Geometry: final body of the model. Coordinates: model frame, mm. Face numbers are marked on the shaded views. A direction names the side the tool comes from. Coordinates: 2 decimals unless noted, no trailing zeros. Order: outer loops, then holes, each group sorted by start corner. A loop starts at its lowest first (then second) coordinate and runs counter-clockwise, first axis right, second up. Notation, with made-up numbers: (45.25, 70) - (66.25, 70) arc R29 ccw to (66.25, 99) - close; hole circle Ø2 at (-25, 39). An arc over 180 degrees is marked (long way). Use a Markdown table: item, result. Add a question column.
```python
from build123d import *

# Parameters (mm, degrees)
EXTRUDE_1_DEPTH     = 5
SKETCH_2_R          = 5
CUT_EXTRUDE_1_DEPTH = 32.721443851
SKETCH_3_W          = 35
SKETCH_3_H          = 35
EXTRUDE_2_DEPTH     = 5
FILLET_1_R          = 10
SKETCH_4_R          = 5
CUT_EXTRUDE_2_DEPTH = 52.780787943


with BuildPart() as part:
    # 草图1 → 凸台-拉伸1 (new body)
    with BuildSketch(Plane.XY):
        with BuildLine():
            Line((0, 20), (0, -20))
            ThreePointArc((0, -20), (-7.5, -27.5), (-15, -20))
            Line((-15, -20), (-15, 20))
            ThreePointArc((-15, 20), (-7.5, 27.5), (0, 20))
        make_face()
    extrude(amount=EXTRUDE_1_DEPTH)

    # 草图2 → 切除-拉伸1 (cut, through all)
    with BuildSketch(Plane.XY.offset(5)):
        with Locations((-7.5, 20)):
            Circle(SKETCH_2_R)
        with Locations((-7.5, -20)):
            Circle(SKETCH_2_R)
    extrude(amount=-CUT_EXTRUDE_1_DEPTH, mode=Mode.SUBTRACT)

    # 草图3 → 凸台-拉伸2 (add, symmetric)
    with BuildSketch(Plane(origin=(0, 0, 0), x_dir=(1, 0, 0), z_dir=(0, 1, 0))):
        with Locations((17.5, -2.5)):
            Rectangle(SKETCH_3_W, SKETCH_3_H)
    extrude(amount=EXTRUDE_2_DEPTH, both=True)

    # 圆角1
    fillet_1_edges = [part.edges().sort_by_distance(p)[0] for p in [
        (0, 0, -15),
        (0, 0, 20),
        (35, 0, 20),
        (35, 0, -15),
    ]]
    fillet(fillet_1_edges, radius=FILLET_1_R)

    # 草图4 → 切除-拉伸2 (cut, through all)
    with BuildSketch(Plane(origin=(0, 5, 0), x_dir=(1, 0, 0), z_dir=(0, 1, 0))):
        with Locations(Location((17.5, -2.5, 0), (0, 0, 270))):
            Circle(SKETCH_4_R)
    extrude(amount=-CUT_EXTRUDE_2_DEPTH, mode=Mode.SUBTRACT)


solid = part.part
```
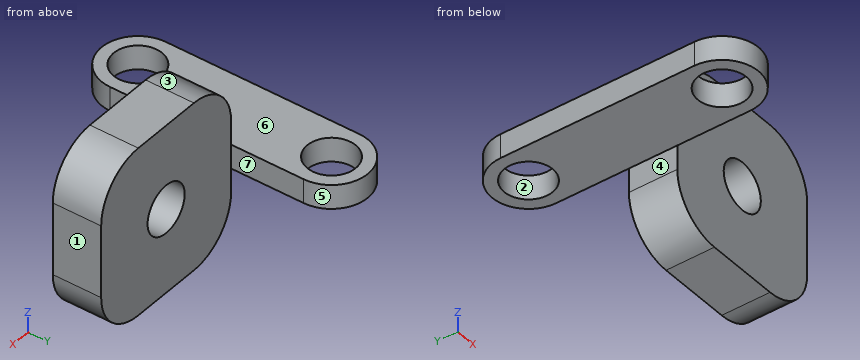
1) Draft query along X for the marked faces 1, 2 and 3. Return one class per face: pulls with the +X half, pulls with the -X half, needs draft (parallel to the pull), parting line crosses it, or undercut.
2) Pin query (flat end, axial travel): pin 1 (5.5 mm diameter, centred on y = -12.5, z = 3.5, fed in from +X); pin 2 (13 mm diameter, centred on x = -7.5, y = 20, fed in from -Z); pin 3 (4 mm diameter, centred on y = -1, z = 8.5, fed in from -X). Return the tip coordinate at first contact, or that it passes through.
3) Section A-A (y = 16). Return loops of the section in (x, z), then the cut area to 3 significant figures.
4) Section C-C (x = 17.5). Return loops of the section in (y, z).
5) Section B-B (x = -7.5). Return loops of the section in (y, z).
6) Set-up query: the marked faces 4, 5, 6 and 7. Return all of +Z, -Z, +X, -X, +Y, -Y with unobstructed straight access to the full face (end or side cutting, diameter ignored); none if empty.
7) Section D-D (y = 0). Return loops of the section in (x, z).
8) Ray query, line 1 along Y through (x, z) = (-7.5, 4); line 2 along Y through (x, z) = (3.5, 5); line 3 along Z through (x, y) = (-5.5, -2). Return the intervals inside material, ascending.
Values follow:
| question | item | result |
|---|---|---|
| 1 | face 1 | pulls with the +X half |
| 1 | face 2 | undercut |
| 1 | face 3 | pulls with the -X half |
| 2 | pin 1 | stops at x = 0 |
| 2 | pin 2 | stops at z = 0 |
| 2 | pin 3 | stops at x = 0 |
| 3 | outline | (-15, 0) - (-10.5, 0) - (-10.5, 5) - (-15, 5) - close; (-4.5, 0) - (0, 0) - (0, 5) - (-4.5, 5) - close |
| 3 | area | 45.0 mm² |
| 4 | outline | (-5, -15) - (5, -15) - (5, -2.5) - (-5, -2.5) - close; (-5, 7.5) - (5, 7.5) - (5, 20) - (-5, 20) - close |
| 5 | outline | (-27.5, 0) - (-25, 0) - (-25, 5) - (-27.5, 5) - close; (-15, 0) - (15, 0) - (15, 5) - (-15, 5) - close; (25, 0) - (27.5, 0) - (27.5, 5) - (25, 5) - close |
| 6 | face 4 | -Z, -X, +Y, -Y |
| 6 | face 5 | +Z, -Z, +Y |
| 6 | face 6 | +Z, -X, +Y, -Y |
| 6 | face 7 | +Z, -Z, +X, +Y |
| 7 | outline | (-15, 0) - (0, 0) - (0, -5) arc R10 ccw to (10, -15) - (25, -15) arc R10 ccw to (35, -5) - (35, 10) arc R10 ccw to (25, 20) - (10, 20) arc R10 ccw to (0, 10) - (0, 5) - (-15, 5) - close; hole circle Ø10 at (17.5, 2.5) |
| 8 | line 1 | y = -27.5 to -25, -15 to 15, 25 to 27.5 |
| 8 | line 2 | y = -5 to 5 |
| 8 | line 3 | z = 0 to 5 |
